Check sheet for the modelled part. Datum: model origin and axes. Units: mm. A direction names the side the tool comes from. Give positions to 0.01 mm unless a question says otherwise; leave off trailing zeros. Write each loop counter-clockwise with the first axis right and the second up, starting at its lowest first coordinate (ties: lowest second). Pieces come first, ordered by that corner, then holes. Notation, with made-up numbers: (11.5, -38) -> (42.5, -38) arc R15 ccw to (42.5, -23) -> close; hole circle Ø7 at (29.5, 51.25). An arc over 180 degrees is marked (long way). Answer as a JSON object with one key per item and string values.
from build123d import *

# Parameters (mm, degrees)
BOSS_EXTRUDE1_DEPTH = 11
SKETCH2_R           = 6
CUT_EXTRUDE1_DEPTH  = 68.666018059
SKETCH3_R           = 2.25
CUT_EXTRUDE2_DEPTH  = 58.635080463
CHAMFER1_SIZE       = 2
CUT_EXTRUDE3_START  = -61.7
SKETCH4_R           = 7.25
CUT_EXTRUDE3_DEPTH  = 59.7


with BuildPart() as part:
    # Sketch1 → Boss-Extrude1 (new, symmetric)
    with BuildSketch(Plane.XY):
        Polygon((-19.25, 20), (-19.25, -20), (44.45, -20), (44.45, 20), (34.45, 20), (34.45, -15), (-9.25, -15), (-9.25, 20), align=None)
    extrude(amount=BOSS_EXTRUDE1_DEPTH, both=True)

    # Sketch2 → Cut-Extrude1 (cut, through all)
    with BuildSketch(Plane(origin=(44.45, 0, 0), x_dir=(0, 0, -1), z_dir=(1, 0, 0))):
        with Locations((0, 9)):
            Circle(SKETCH2_R)
        with BuildLine():
            Line((-11, 9), (-11, 20))
            Line((-11, 20), (-11, 31))
            Line((-11, 31), (11, 31))
            Line((11, 31), (11, 20))
            Line((11, 20), (11, 9))
            ThreePointArc((11, 9), (7.778174593, 16.778174593), (0, 20))
            ThreePointArc((0, 20), (-7.778174593, 16.778174593), (-11, 9))
        make_face()
    extrude(amount=-CUT_EXTRUDE1_DEPTH, mode=Mode.SUBTRACT)

    # Sketch3 → Cut-Extrude2 (cut, through all)
    with BuildSketch(Plane(origin=(0, -15, 0), x_dir=(1, 0, 0), z_dir=(0, 1, 0))):
        with Locations(Location((0, 5.75, 0), (0, 0, 270))):
            Circle(SKETCH3_R)
        with Locations(Location((0, -5.75, 0), (0, 0, 270))):
            Circle(SKETCH3_R)
        with Locations(Location((25.2, 5.75, 0), (0, 0, 270))):
            Circle(SKETCH3_R)
        with Locations(Location((25.2, -5.75, 0), (0, 0, 270))):
            Circle(SKETCH3_R)
    extrude(amount=-CUT_EXTRUDE2_DEPTH, mode=Mode.SUBTRACT)

    # Chamfer1
    chamfer1_edges = [part.edges().sort_by_distance(p)[0] for p in [
        (0, -15, 3.5),
        (25.2, -15, -8),
        (25.2, -15, 3.5),
        (0, -15, -8),
    ]]
    chamfer(chamfer1_edges, length=CHAMFER1_SIZE)

    # Sketch4 → Cut-Extrude3 (cut)
    with BuildSketch(Plane(origin=(44.45, 0, 0), x_dir=(0, 0, -1), z_dir=(1, 0, 0)).offset(CUT_EXTRUDE3_START)):
        with Locations((0, 9)):
            Circle(SKETCH4_R)
    extrude(amount=CUT_EXTRUDE3_DEPTH, mode=Mode.SUBTRACT)


solid = part.part
1. Mould release check, pull along X, two halves, no side actions. Record for faces 4 (the face through (-19.25, -4, 0)), 5 (the face through (42.45, 15, 2)), 6 (the face through (12, -16, -11)): released by +X, released by -X, zero draft, split by the parting line, or undercut.
Determined:
{"face 4": "released by -X", "face 5": "undercut", "face 6": "zero draft"}
2. Scan lines: L1, parallel to X at y = 11, z = -8.25; L2, parallel to Z at x = 40.75, y = 9; L3, parallel to Y at x = 39.5, z = 0. Record each from-to range of solid material in increasing order. Write a range as [from, to].
Determined:
{"L1": "[-19.25, -9.25], [34.45, 44.45]", "L2": "[-11, -7.25], [7.25, 11]", "L3": "[-20, 1.75], [16.25, 20]"}
3. Sectioned sample at B-B, the plane x = -12. Enter the section's corners in (y, z), plus the area to 3 significant figures.
Determined:
{"outline": "(-20, -11) -> (9, -11) arc R11 ccw to (9, 11) -> (-20, 11) -> close; hole circle Ø14.5 at (9, 0)", "area": "663 mm^2"}
4. Sectioned sample at A-A, the plane y = -9. Enter the section's corners in (x, z).
Determined:
{"outline": "(-19.25, -11) -> (-9.25, -11) -> (-9.25, 11) -> (-19.25, 11) -> close; (34.45, -11) -> (44.45, -11) -> (44.45, 11) -> (34.45, 11) -> close"}
5. Sectioned sample at C-C, the plane y = 12. Enter the section's corners in (x, z), plus the area to 3 significant figures.
Determined:
{"outline": "(-19.25, -10.58) -> (-9.25, -10.58) -> (-9.25, -6.6) -> (-17.25, -6.6) -> (-17.25, -5.2) -> (-19.25, -5.2) -> close; (-19.25, 5.2) -> (-17.25, 5.2) -> (-17.25, 6.6) -> (-9.25, 6.6) -> (-9.25, 10.58) -> (-19.25, 10.58) -> close; (34.45, -10.58) -> (44.45, -10.58) -> (44.45, -5.2) -> (42.45, -5.2) -> (42.45, -6.6) -> (34.45, -6.6) -> close; (34.45, 6.6) -> (42.45, 6.6) -> (42.45, 5.2) -> (44.45, 5.2) -> (44.45, 10.58) -> (34.45, 10.58) -> close", "area": "171 mm^2"}
6. Go/stop test with flat-tipped pins: P1, Ø4, axis at x = 0, z = 5.75, coming from the +Y side; P2, Ø11, axis at x = 2, z = -0.5, coming from the +Y side; P3, Ø10, axis at x = -9.5, z = 7.5, coming from the +Y side; P4, Ø7, axis at x = 25.2, z = -5.75, coming from the +Y side. Record where each tip stops, or that it passes through.
Determined:
{"P1": "through", "P2": "y = -15", "P3": "y = 19.71", "P4": "y = -15.75"}
7. Sectioned sample at D-D, the plane x = 32. Enter the section's corners in (y, z), plus the area to 3 significant figures.
Determined:
{"outline": "(-20, -11) -> (-15, -11) -> (-15, 11) -> (-20, 11) -> close", "area": "110 mm^2"}
8. Access from +Z, -Z, +X, -X, +Y, -Y to the whole of each face (thin tool, end or side, straight path). Record for faces 1 (the face through (-17.25, 15, 2)), 2 (the face through (23.204, -18.479, 6.788)), 3 (the face through (34.45, -1, 0)).
Determined:
{"face 1": "none", "face 2": "+Y, -Y", "face 3": "+Z, -Z, +Y"}
